from build123d import *

# Parameters (mm, degrees)
SKETCH1_R           = 38.1
BOSS_EXTRUDE1_DEPTH = 365.76
SKETCH2_W           = 15.24
SKETCH2_H           = 15.24
CUT_EXTRUDE1_DEPTH  = 304.8
SKETCH3_W           = 15.24
SKETCH3_H           = 15.24
CUT_EXTRUDE2_DEPTH  = 12.7


with BuildPart() as part:
    # Sketch1 → Boss-Extrude1 (new body)
    with BuildSketch(Plane(origin=(0, 0, 0), x_dir=(0, 0, -1), z_dir=(1, 0, 0))):
        Circle(SKETCH1_R)
    extrude(amount=BOSS_EXTRUDE1_DEPTH)

    # Sketch2 → Cut-Extrude1 (cut)
    with BuildSketch(Plane(origin=(365.76, 0, 0), x_dir=(0, 0, -1), z_dir=(1, 0, 0))):
        with Locations((0, 38.1)):
            Rectangle(SKETCH2_W, SKETCH2_H)
    extrude(amount=-CUT_EXTRUDE1_DEPTH, mode=Mode.SUBTRACT)

    # Sketch3 → Cut-Extrude2 (cut)
    with BuildSketch(Plane.ZY):
        with Locations((0, 38.1)):
            Rectangle(SKETCH3_W, SKETCH3_H)
    extrude(amount=-CUT_EXTRUDE2_DEPTH, mode=Mode.SUBTRACT)


solid = part.part
Can you work these out from the model? Positions are in its coordinate system, mm. A direction names the side the tool comes from. Give positions to 0.01 mm unless a question says otherwise; leave off trailing zeros. Order: outer loops, then holes, each group sorted by start corner. A loop starts at its lowest first (then second) coordinate and runs counter-clockwise, first axis right, second up. Notation, with made-up numbers: M 48.5,-37.75 L 86.5,-37.75 A29 ccw 86.5,-0.75 Z; hole C -28.5,57.25 d3. An arc over 180 degrees is marked long. Use one line per item in the form item = value. Start each with the question number.
Item 1: For faces 4 (the flat face through (0, 0, 1)), 5 (the flat face through (215, 34, 7.62)), 6 (the flat face through (6, 34, -7.62)), which set-ups out of +Z, -Z, +X, -X, +Y, -Y let a thin tool reach every point of the face, with its end or its side?
Item 2: If we section it at B-B (x = 296.5): Write out the boundary of the cut face in (y, z).
Item 3: If we section it at C-C (y = 22.5): Write out the boundary of the cut face in (x, z), then the cut area to 3 significant figures.
Item 4: If I drill on line 1 along Z through (x, y) = (236, 34); line 2 along Y through (x, z) = (35, 20); line 3 along Z through (x, y) = (77, 2), over which ranges is the centre line in solid material (lowest first)?
Item 5: Will these pins go through, and if not, where does the flat tip stop? pin 1 Ø7.5 at (x, z) = (220.5, -2) entering from +Y; pin 2 Ø1 at (x, y) = (118, 7) entering from -Z; pin 3 Ø2 at (y, z) = (9, -26.5) entering from -X; pin 4 Ø7.5 at (x, y) = (177, 32.5) entering from +Z.
Item 6: If we section it at A-A (z = 0): Write out the boundary of the cut face in (x, y), then the cut area to 3 significant figures.
Item 7: We'd pull the mould along Z, two halves only. Please class faces 1 (the flat face through (215, 30.48, 0)), 2 (the cylindrical face through (180.32, -37.194, 8.259)), 3 (the flat face through (365.76, 0, 1)): +Z half, -Z half, draft (parallel to the pull), parting line (faces both ways), or undercut.
Outcome:
q1.face_4 = +Z, -Z, -X, +Y, -Y
q1.face_5 = +X, +Y
q1.face_6 = -X, +Y
q2.outline = M 30.48,-7.62 L 30.48,7.62 L 37.33,7.62 A38.1 ccw long 37.33,-7.62 Z
q3.outline = M 0,-30.75 L 365.76,-30.75 L 365.76,30.75 L 0,30.75 Z
q3.area = 22,500 mm2
q4.line_1 = -17.19 to -7.62, 7.62 to 17.19
q4.line_2 = -32.43 to 32.43
q4.line_3 = -38.05 to 38.05
q5.pin_1 = 30.48
q5.pin_2 = -37.54
q5.pin_3 = 0
q5.pin_4 = 25
q6.outline = M 0,-38.1 L 365.76,-38.1 L 365.76,30.48 L 60.96,30.48 L 60.96,38.1 L 12.7,38.1 L 12.7,30.48 L 0,30.48 Z
q6.area = 25,500 mm2
q7.face_1 = undercut
q7.face_2 = parting line
q7.face_3 = draft
